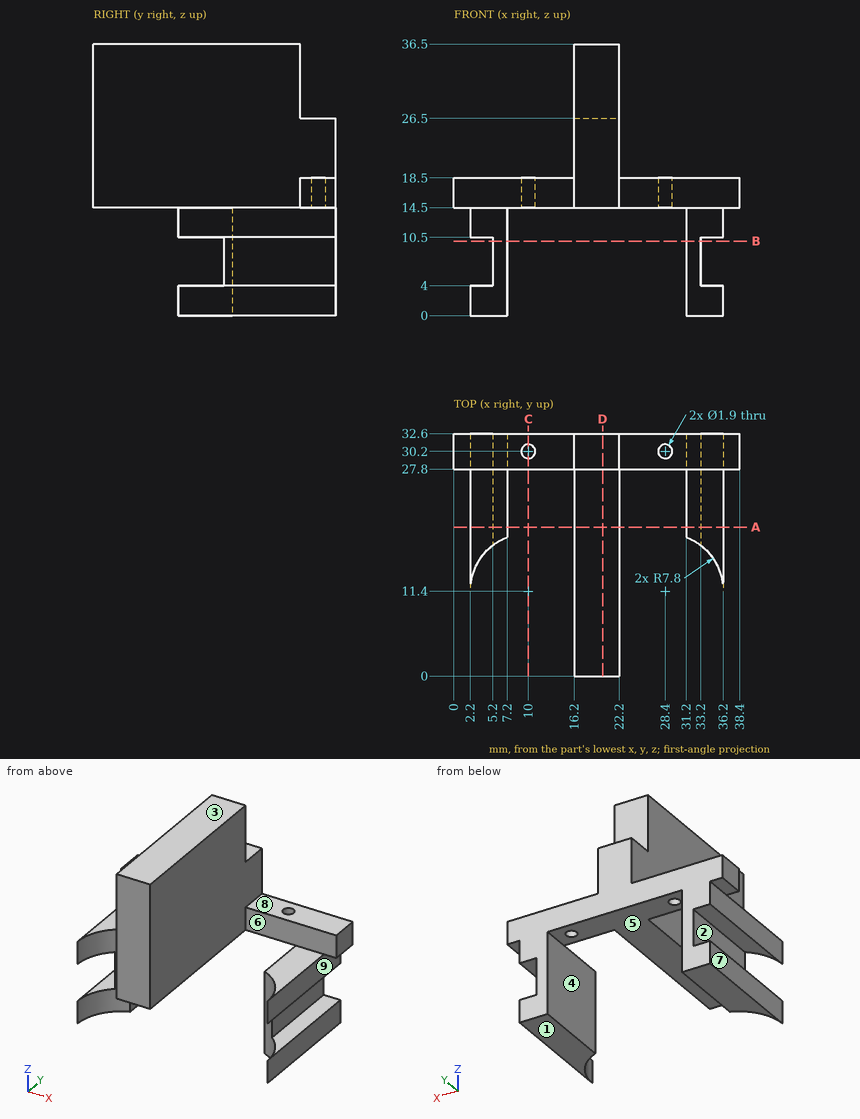
Check sheet for the drawn part. Datum: minimum x, y, z corner. Units: mm. A direction names the side the tool comes from. Give positions to 0.01 mm unless a question says otherwise; leave off trailing zeros. Order: outer loops, then holes, each group sorted by start corner. A loop starts at its lowest first (then second) coordinate and runs counter-clockwise, first axis right, second up. Notation, with made-up numbers: (16, -23) -> (37, -23) arc R20 ccw to (37, 12) -> close; hole circle Ø3 at (17, 43.5). An arc over 180 degrees is marked (long way). Return JSON: item names as keys, results as strings.
1. Set-up check for the marked faces 5, 6, 7, 8 and 9: record each of +Z, -Z, +X, -X, +Y, -Y from which the full face is reachable in a straight line by a thin tool's end or side.
From the geometry:
{"face 5": "-Z, +Y, -Y", "face 6": "+Z, +X, -Y", "face 7": "-Z, -X, +Y, -Y", "face 8": "+Z, +X, +Y, -Y", "face 9": "-Z, +X, +Y, -Y"}
2. Material ranges on probe 1 along Z at (x, y) = (3.5, 24.5); probe 2 along Y at (x, z) = (10, 17); probe 3 along X at (y, z) = (27, 5), recorded low to high. Write a range as [from, to].
From the geometry:
{"probe 1": "[0, 4], [10.5, 14.5]", "probe 2": "[27.8, 29.25], [31.15, 32.6]", "probe 3": "[5.2, 7.2], [31.2, 33.2]"}
3. Cross-section at D-D, the plane x = 20. Record the cut outline in (y, z), plus the area to 3 significant figures.
From the geometry:
{"outline": "(0, 14.5) -> (32.6, 14.5) -> (32.6, 26.5) -> (27.8, 26.5) -> (27.8, 36.5) -> (0, 36.5) -> close", "area": "669 mm^2"}
4. Cross-section at A-A, the plane y = 20. Record the cut outline in (x, z), plus the area to 3 significant figures.
From the geometry:
{"outline": "(2.2, 0) -> (7.2, 0) -> (7.2, 14.5) -> (2.2, 14.5) -> (2.2, 10.5) -> (5.2, 10.5) -> (5.2, 4) -> (2.2, 4) -> close; (16.2, 14.5) -> (22.2, 14.5) -> (22.2, 36.5) -> (16.2, 36.5) -> close; (31.2, 0) -> (36.2, 0) -> (36.2, 4) -> (33.2, 4) -> (33.2, 10.5) -> (36.2, 10.5) -> (36.2, 14.5) -> (31.2, 14.5) -> close", "area": "238 mm^2"}
5. Go/stop test with flat-tipped pins: P1, Ø2.5, axis at x = 28.4, y = 30.2, coming from the +Z side; P2, Ø10, axis at x = 6, z = 6.5, coming from the -Y side; P3, Ø12, axis at y = 18, z = 31, coming from the +X side; P4, Ø1.7, axis at x = 10, y = 30.2, coming from the -Z side. Record where each tip stops, or that it passes through.
From the geometry:
{"P1": "z = 18.5", "P2": "y = 11.4", "P3": "x = 22.2", "P4": "through"}
6. Mould release check, pull along Z, two halves, no side actions. Record for the marked faces 1, 2, 3 and 4: +Z half, -Z half, draft (parallel to the pull), parting line (faces both ways), or undercut.
From the geometry:
{"face 1": "-Z half", "face 2": "undercut", "face 3": "+Z half", "face 4": "draft"}
7. Cross-section at C-C, the plane x = 10. Record the cut outline in (y, z).
From the geometry:
{"outline": "(27.8, 14.5) -> (29.25, 14.5) -> (29.25, 18.5) -> (27.8, 18.5) -> close; (31.15, 14.5) -> (32.6, 14.5) -> (32.6, 18.5) -> (31.15, 18.5) -> close"}
8. Cross-section at B-B, the plane z = 10. Record the cut outline in (x, y).
From the geometry:
{"outline": "(5.2, 17.55) arc R7.8 cw to (7.2, 18.68) -> (7.2, 32.6) -> (5.2, 32.6) -> close; (31.2, 18.68) arc R7.8 cw to (33.2, 17.55) -> (33.2, 32.6) -> (31.2, 32.6) -> close"}
